Check sheet for the modelled part. Datum: model origin and axes. Units: mm. A direction names the side the tool comes from. Round coordinates to 2 decimals unless told otherwise and drop trailing zeros. Write each loop counter-clockwise with the first axis right and the second up, starting at its lowest first coordinate (ties: lowest second). Pieces come first, ordered by that corner, then holes. Notation, with made-up numbers: (70, 87.5) -> (86, 87.5) arc R23 ccw to (86, 111.5) -> close; hole circle Ø10 at (47.25, -18.5). An arc over 180 degrees is marked (long way). One line per item, written item: value.
Autodesk Inventor part; units mm, degrees
ref_plane "YZ Plane" through (0, 0, 0) normal (1, 0, 0) x (0, 1, 0)
ref_plane "XZ Plane" through (0, 0, 0) normal (0, 1, 0) x (-1, 0, 0)
ref_plane "XY Plane" through (0, 0, 0) normal (0, 0, 1) x (1, 0, 0)
sketch "Sketch1" plane through (0, 0, 0) normal (0, 1, 0) x (-1, 0, 0)
  line L0 (45, -30) -> (-45, -30)
  line L1 (-45, -30) -> (-45, 30)
  line L2 (-45, 30) -> (45, 30)
  line L3 (45, 30) -> (45, -30)
  line L4 (45, -30) -> (-45, 30) construction
  line L5 (-45, -30) -> (45, 30) construction
  line L6 (30, -30) -> (-30, -30)
  line L7 (-30, -30) -> (-30, 30)
  line L8 (-30, 30) -> (30, 30)
  line L9 (30, 30) -> (30, -30)
  line L10 (30, -30) -> (-30, 30) construction
  line L11 (-30, -30) -> (30, 30) construction
  point P0 (0, 0)
  point P1 (30, -30)
  point P2 (30, 30)
  dimension "d0" = 90
  dimension "d1" = 60
  dimension "d2" = 60
extrude "Extrusion1" add sketch "Sketch1" against normal blind 10 contours L0 L7 L2 L9
extrude "Extrusion2" add sketch "Sketch1" along normal blind 80 and the other way blind 10 contours L0 L9 L2 L3 | L0 L1 L2 L7
sketch "Sketch3" plane through (0, -10, 0) normal (0, -1, 0) x (1, 0, 0)
  point P0 (0, 0)
  point P1 (0, 5)
  point P2 (0, -5)
  dimension "d16" = 5
  dimension "d17" = 5
hole "Hole2" at (0, -10, 5) at (0, -10, -5) direction (0, 1, 0) diameter 5.5 end through all
sketch "Sketch4" plane through (45, -10, -30) normal (1, 0, 0) x (0, 0, -1)
  circle A0 centre (-30, 65) radius 11
  line L0 (-41, 65) -> (-41, 90)
  line L1 (-60, 90) -> (0, 90)
  line L2 (-19, 65) -> (-19, 90)
  circle A1 centre (-30, 65) radius 7.5
  point P0 (-30, 10)
  dimension "d25" = 22
  dimension "d26" = 15
  dimension "d27" = 25
extrude "Extrusion3" cut sketch "Sketch4" against normal through all contours A1
sketch "Sketch5" plane through (0, 80, 0) normal (0, 1, 0) x (1, 0, 0)
  line L0 (-41.5, 11.25) -> (-33.5, 11.25)
  line L1 (-33.5, 11.25) -> (-33.5, -11.25)
  line L2 (-33.5, -11.25) -> (-41.5, -11.25)
  line L3 (-41.5, -11.25) -> (-41.5, 11.25)
  line L4 (-41.5, 11.25) -> (-33.5, -11.25) construction
  line L5 (-33.5, 11.25) -> (-41.5, -11.25) construction
  line L6 (33.5, 11.25) -> (41.5, 11.25)
  line L7 (41.5, 11.25) -> (41.5, -11.25)
  line L8 (41.5, -11.25) -> (33.5, -11.25)
  line L9 (33.5, -11.25) -> (33.5, 11.25)
  line L10 (33.5, 11.25) -> (41.5, -11.25) construction
  line L11 (41.5, 11.25) -> (33.5, -11.25) construction
  line L12 (-45, 30) -> (-45, -30)
  line L13 (-30, 30) -> (-45, 30)
  line L14 (45, 30) -> (30, 30)
  point P0 (0, 0)
  point P1 (-37.5, 0)
  point P2 (37.5, 0)
  point P3 (-37.5, 0)
  point P4 (37.5, 0)
  point P5 (-37.5, 0)
  point P6 (-45, 0)
  point P7 (-37.5, 30)
  point P8 (-37.5, 11.25)
  point P9 (37.5, 11.25)
  point P10 (37.5, 30)
  dimension "d32" = 8
  dimension "d33" = 22.5
  dimension "d34" = 8
  dimension "d35" = 22.5
extrude "Extrusion5" cut sketch "Sketch5" against normal blind 36.75
sketch "Sketch6" plane through (45, -10, -30) normal (1, 0, 0) x (0, 0, -1)
  point P0 (-30, 10)
sketch "Sketch7" plane through (-45, -10, 30) normal (-1, 0, 0) x (0, 0, 1)
  line L0 (-69.6025, -105.0508) -> (27.4472, -105.0508)
  line L1 (27.4472, -105.0508) -> (27.4472, 137.5734)
  line L2 (27.4472, 137.5734) -> (-69.6025, 137.5734)
  line L3 (-69.6025, 137.5734) -> (-69.6025, -105.0508)
  point P0 (-30, 10)
extrude "Extrusion6" cut sketch "Sketch7" against normal up to surface (75 mm away)
sketch "Sketch8" plane through (0, -10, 0) normal (0, -1, 0) x (1, 0, 0)
  line L0 (55.2414, 58.8952) -> (10.7003, 58.8952)
  line L1 (10.7003, 58.8952) -> (10.7003, -57.3293)
  line L2 (10.7003, -57.3293) -> (55.2414, -57.3293)
  line L3 (55.2414, -57.3293) -> (55.2414, 58.8952)
  point P0 (0, 0)
extrude "Extrusion7" cut sketch "Sketch8" against normal blind 30
sketch "Sketch9" plane through (0, 20, 0) normal (0, -1, 0) x (1, 0, 0)
  line L0 (45, -30) -> (30, -30)
  line L1 (30, 30) -> (45, 30)
  point P0 (0, 0)
  point P1 (37.5, 15)
  point P2 (37.5, -15)
  point P3 (37.5, -30)
  dimension "d45" = 15
  dimension "d46" = 15
hole "Hole3" at (37.5, 20, 15) at (37.5, 20, -15) direction (0, 1, 0) diameter 4.134 end through all
equation "\"d34\" = d32"
equation "\"d35\" = d33"
properties part number "Soporte_Horizontal_Modificado" material "ABS Plastic"
Item 1: Sectioned sample at B-B on z = 0. Enter the section's corners in (x, y), and give its area (3 significant figures).
Answer:
outline: (30, 20) -> (45, 20) -> (45, 47.5) -> (41.5, 47.5) -> (41.5, 43.25) -> (33.5, 43.25) -> (33.5, 47.5) -> (30, 47.5) -> close; (30, 62.5) -> (33.5, 62.5) -> (33.5, 80) -> (30, 80) -> close; (41.5, 62.5) -> (45, 62.5) -> (45, 80) -> (41.5, 80) -> close
area: 501 mm^2
Item 2: Sectioned sample at C-C on x = 37.5. Enter the section's corners in (y, z), and give its area (3 significant figures).
Answer:
outline: (20, -30) -> (80, -30) -> (80, -17.07) -> (20, -17.07) -> close; (20, -12.93) -> (80, -12.93) -> (80, -11.25) -> (43.25, -11.25) -> (43.25, 11.25) -> (80, 11.25) -> (80, 12.93) -> (20, 12.93) -> close; (20, 17.07) -> (80, 17.07) -> (80, 30) -> (20, 30) -> close
area: 2,280 mm^2
Item 3: Sectioned sample at A-A on y = 55. Enter the section's corners in (x, z), and give its area (3 significant figures).
Answer:
outline: (30, -30) -> (45, -30) -> (45, -7.5) -> (41.5, -7.5) -> (41.5, -11.25) -> (33.5, -11.25) -> (33.5, -7.5) -> (30, -7.5) -> close; (30, 7.5) -> (33.5, 7.5) -> (33.5, 11.25) -> (41.5, 11.25) -> (41.5, 7.5) -> (45, 7.5) -> (45, 30) -> (30, 30) -> close; hole circle Ø4.13 at (37.5, -15); hole circle Ø4.13 at (37.5, 15)
area: 588 mm^2
Item 4: Mould release check, pull along Y, two halves, no side actions. Record for faces 1 (the flat face through (37, 20, 0)), 2 (the flat face through (30, 43, 0)), 3 (the cylindrical face through (31.77, 47.68, 1.63)), 4 (the cylindrical face through (43.27, 47.68, 1.63)): pulls with the +Y half, pulls with the -Y half, needs draft (parallel to the pull), parting line crosses it, or undercut.
Answer:
face 1: pulls with the -Y half
face 2: needs draft
face 3: undercut
face 4: undercut
Item 5: Depth check by flat-ended pin: P1, Ø2.5, axis at x = 37, z = 2, coming from the +Y side. Enter the tip coordinate at first touch or a pass-through.
Answer:
P1: stops at y = 43.25
Item 6: Tool access check on faces 5 (the flat face through (38, 50, 30)), 6 (the flat face through (37, 43.25, 0)). Record the directions out of +Z, -Z, +X, -X, +Y, -Y that give a thin tool (end or side, any length) a straight path to the whole face; none if there is none.
Answer:
face 5: +Z, +X, -X, +Y, -Y
face 6: +Y
Item 7: Sectioned sample at D-D on y = 71. Enter the section's corners in (x, z).
Answer:
outline: (30, -30) -> (45, -30) -> (45, 30) -> (30, 30) -> close; hole (33.5, -11.25) -> (41.5, -11.25) -> (41.5, 11.25) -> (33.5, 11.25) -> close; hole circle Ø4.13 at (37.5, -15); hole circle Ø4.13 at (37.5, 15)
Item 8: Thickness scan on line 1 (Z direction, x = 37.5, y = 66); line 2 (Y direction, x = 44.3, z = 0); line 3 (Z direction, x = 37.5, y = 42.5). Record the ranges inside material, lowest first.
Answer:
line 1: z = -30 to -17.07, -12.93 to -11.25, 11.25 to 12.93, 17.07 to 30
line 2: y = 20 to 47.5, 62.5 to 80
line 3: z = -30 to -17.07, -12.93 to 12.93, 17.07 to 30
